Verification items for the finished model (mm, model axes). A direction names the side the tool comes from. Round coordinates to 2 decimals unless told otherwise and drop trailing zeros. Write each loop counter-clockwise with the first axis right and the second up, starting at its lowest first coordinate (ties: lowest second). Pieces come first, ordered by that corner, then holes.
from build123d import *

# Parameters (mm, degrees)
BOSS_EXTRUDE1_START = 0.2
BOSS_EXTRUDE1_DEPTH = 2.3
BOSS_EXTRUDE2_DEPTH = 1.5
SKETCH3_R           = 1.55
CUT_EXTRUDE1_DEPTH  = 25.009164917
CHAMFER1_SIZE       = 0.7
FILLET1_R           = 0.6
SKETCH4_R           = 2.7
CUT_EXTRUDE2_DEPTH  = 1
BOSS_EXTRUDE3_START = 0.3
BOSS_EXTRUDE3_DEPTH = 0.3


with BuildPart() as part:
    # Sketch1 → Boss-Extrude1 (new body)
    with BuildSketch(Plane(origin=(0, 0, 0), x_dir=(1, 0, 0), z_dir=(0, 1, 0)).offset(BOSS_EXTRUDE1_START)):
        with BuildLine():
            Line((5.6, -14.5), (5.6, 14.5))
            ThreePointArc((5.6, 14.5), (5.277817459, 15.277817459), (4.5, 15.6))
            Line((4.5, 15.6), (-4.5, 15.6))
            ThreePointArc((-4.5, 15.6), (-5.277817459, 15.277817459), (-5.6, 14.5))
            Line((-5.6, 14.5), (-5.6, -14.5))
            ThreePointArc((-5.6, -14.5), (-5.277817459, -15.277817459), (-4.5, -15.6))
            Line((-4.5, -15.6), (4.5, -15.6))
            ThreePointArc((4.5, -15.6), (5.277817459, -15.277817459), (5.6, -14.5))
        make_face()
    extrude(amount=BOSS_EXTRUDE1_DEPTH)

    # Sketch2 → Boss-Extrude2 (add)
    with BuildSketch(Plane(origin=(0, 2.5, 0), x_dir=(1, 0, 0), z_dir=(0, 1, 0))):
        with BuildLine():
            Line((-4.5, -21), (4.5, -21))
            ThreePointArc((4.5, -21), (9.096194078, -19.096194078), (11, -14.5))
            Line((11, -14.5), (11, 14.5))
            ThreePointArc((11, 14.5), (9.096194078, 19.096194078), (4.5, 21))
            Line((4.5, 21), (-4.5, 21))
            ThreePointArc((-4.5, 21), (-9.096194078, 19.096194078), (-11, 14.5))
            Line((-11, 14.5), (-11, -14.5))
            ThreePointArc((-11, -14.5), (-9.096194078, -19.096194078), (-4.5, -21))
        make_face()
    extrude(amount=BOSS_EXTRUDE2_DEPTH)

    # Sketch3 → Cut-Extrude1 (cut, through all)
    with BuildSketch(Plane(origin=(0, 4, 0), x_dir=(1, 0, 0), z_dir=(0, 1, 0))):
        with Locations(Location((3.05, -13.05, 0), (0, 0, 270))):
            Circle(SKETCH3_R)
        with Locations(Location((3.05, 13.05, 0), (0, 0, 270))):
            Circle(SKETCH3_R)
        with Locations(Location((-3.05, 13.05, 0), (0, 0, 270))):
            Circle(SKETCH3_R)
        with Locations(Location((-3.05, -13.05, 0), (0, 0, 270))):
            Circle(SKETCH3_R)
    extrude(amount=-CUT_EXTRUDE1_DEPTH, mode=Mode.SUBTRACT)

    # Chamfer1
    chamfer1_edges = [part.edges().sort_by_distance(p)[0] for p in [
        (-11, 4, 0),
        (-9.096194078, 4, 19.096194078),
        (0, 4, 21),
        (9.096194078, 4, 19.096194078),
        (11, 4, 0),
        (9.096194078, 4, -19.096194078),
        (0, 4, -21),
        (-9.096194078, 4, -19.096194078),
    ]]
    chamfer(chamfer1_edges, length=CHAMFER1_SIZE)

    # Fillet1
    fillet1_edges = [part.edges().sort_by_distance(p)[0] for p in [
        (0, 0.2, -15.6),
        (5.277817459, 0.2, -15.277817459),
        (5.6, 0.2, 0),
        (5.277817459, 0.2, 15.277817459),
        (0, 0.2, 15.6),
        (-5.277817459, 0.2, 15.277817459),
        (-5.6, 0.2, 0),
        (-5.277817459, 0.2, -15.277817459),
    ]]
    fillet(fillet1_edges, radius=FILLET1_R)

    # Sketch4 → Cut-Extrude2 (cut)
    with BuildSketch(Plane(origin=(0, 4, 0), x_dir=(1, 0, 0), z_dir=(0, 1, 0))):
        with Locations(Location((-3.05, 13.05, 0), (0, 0, 270))):
            Circle(SKETCH4_R)
        with Locations(Location((3.05, 13.05, 0), (0, 0, 270))):
            Circle(SKETCH4_R)
        with Locations(Location((-3.05, -13.05, 0), (0, 0, 270))):
            Circle(SKETCH4_R)
        with Locations(Location((3.05, -13.05, 0), (0, 0, 270))):
            Circle(SKETCH4_R)
    extrude(amount=-CUT_EXTRUDE2_DEPTH, mode=Mode.SUBTRACT)

    # Sketch5 → Boss-Extrude3 (add)
    with BuildSketch(Plane(origin=(0, 3, 0), x_dir=(1, 0, 0), z_dir=(0, 1, 0)).offset(BOSS_EXTRUDE3_START)):
        with BuildLine():
            Line((4.6, 15.260769097), (4.6, 10.839230903))
            ThreePointArc((4.6, 10.839230903), (5.75, 13.05), (4.6, 15.260769097))
        make_face()
        with BuildLine():
            Line((1.5, 15.260769097), (1.5, 10.839230903))
            ThreePointArc((1.5, 10.839230903), (0.35, 13.05), (1.5, 15.260769097))
        make_face()
        with BuildLine():
            Line((-4.6, 15.260769097), (-4.6, 10.839230903))
            ThreePointArc((-4.6, 10.839230903), (-5.75, 13.05), (-4.6, 15.260769097))
        make_face()
        with BuildLine():
            Line((-1.5, 15.260769097), (-1.5, 10.839230903))
            ThreePointArc((-1.5, 10.839230903), (-0.35, 13.05), (-1.5, 15.260769097))
        make_face()
        with BuildLine():
            Line((-4.6, -10.839230903), (-4.6, -15.260769097))
            ThreePointArc((-4.6, -15.260769097), (-5.75, -13.05), (-4.6, -10.839230903))
        make_face()
        with BuildLine():
            Line((-1.5, -10.839230903), (-1.5, -15.260769097))
            ThreePointArc((-1.5, -15.260769097), (-0.35, -13.05), (-1.5, -10.839230903))
        make_face()
        with BuildLine():
            Line((1.5, -10.839230903), (1.5, -15.260769097))
            ThreePointArc((1.5, -15.260769097), (0.35, -13.05), (1.5, -10.839230903))
        make_face()
        with BuildLine():
            Line((4.6, -10.839230903), (4.6, -15.260769097))
            ThreePointArc((4.6, -15.260769097), (5.75, -13.05), (4.6, -10.839230903))
        make_face()
    extrude(amount=-BOSS_EXTRUDE3_DEPTH)


solid = part.part
Q1. Depth check by flat-ended pin: P1, Ø3, axis at x = -2.5, z = -14, coming from the +Y side; P2, Ø2, axis at x = -3.5, z = 12, coming from the +Y side; P3, Ø0.5, axis at y = 1.5, z = 0, coming from the +X side. Enter the tip coordinate at first touch or a pass-through.
Recorded:
P1: stops at y = 3.3
P2: stops at y = 3
P3: stops at x = 5.6
Q2. Sectioned sample at A-A (x = -3.05). Enter the section's corners in (y, z).
Recorded:
outline: (0.2, -15) arc R0.6 ccw to (0.8, -15.6) - (2.5, -15.6) - (2.5, -21) - (3.3, -21) - (4, -20.3) - (4, -15.75) - (3, -15.75) - (3, -14.6) - (0.2, -14.6) - close; (0.2, -11.5) - (3, -11.5) - (3, -10.35) - (4, -10.35) - (4, 10.35) - (3, 10.35) - (3, 11.5) - (0.2, 11.5) - close; (0.2, 14.6) - (3, 14.6) - (3, 15.75) - (4, 15.75) - (4, 20.3) - (3.3, 21) - (2.5, 21) - (2.5, 15.6) - (0.8, 15.6) arc R0.6 ccw to (0.2, 15) - close
Q3. Sectioned sample at D-D (z = -13.5). Give the number of separate pieces and of enclosed holes in the cut face, plus the area to 3 significant figures.
Recorded:
separate pieces: 3
enclosed holes: 0
area: 32.2 mm2
Q4. Material ranges on line 1 along Z through (x, y) = (3.05, 2.2); line 2 along X through (y, z) = (0.8, -13.05); line 3 along Z through (x, y) = (3.05, 3.3), recorded low to high.
Recorded:
line 1: z = -15.6 to -14.6, -11.5 to 11.5, 14.6 to 15.6
line 2: x = -5.6 to -4.6, -1.5 to 1.5, 4.6 to 5.6
line 3: z = -21 to -15.75, -10.35 to 10.35, 15.75 to 21
Q5. Tool access check on faces 1 (the flat face through (-5.6, 2, 0)), 2 (the cylindrical face through (-5.286, 1.638, 15.269)), 3 (the cylindrical face through (-5.269, 1.638, -15.286)), 4 (the cylindrical face through (-2.239, 3.618, -10.475)), 5 (the flat face through (0, 2, 15.6)). Record the directions out of +Z, -Z, +X, -X, +Y, -Y that give a thin tool (end or side, any length) a straight path to the whole face; none if there is none.
Recorded:
face 1: +Z, -Z, -X, -Y
face 2: +Z, -X, -Y
face 3: -Z, -X, -Y
face 4: +Y
face 5: +Z, +X, -X, -Y
Q6. Sectioned sample at B-B (y = 1.5). Enter the section's corners in (x, z), plus the area to 3 significant figures.
Recorded:
outline: (-5.6, -14.5) arc R1.1 ccw to (-4.5, -15.6) - (4.5, -15.6) arc R1.1 ccw to (5.6, -14.5) - (5.6, 14.5) arc R1.1 ccw to (4.5, 15.6) - (-4.5, 15.6) arc R1.1 ccw to (-5.6, 14.5) - close; hole circle Ø3.1 at (-3.05, -13.05); hole circle Ø3.1 at (-3.05, 13.05); hole circle Ø3.1 at (3.05, -13.05); hole circle Ø3.1 at (3.05, 13.05)
area: 318 mm2
Q7. Sectioned sample at C-C (z = -6.5). Enter the section's corners in (x, y).
Recorded:
outline: (-11, 2.5) - (-5.6, 2.5) - (-5.6, 0.8) arc R0.6 ccw to (-5, 0.2) - (5, 0.2) arc R0.6 ccw to (5.6, 0.8) - (5.6, 2.5) - (11, 2.5) - (11, 3.3) - (10.3, 4) - (-10.3, 4) - (-11, 3.3) - close
